```python
from build123d import *

# Parameters (mm, degrees)
SKETCH1_W                   = 72
SKETCH1_H                   = 35
BOSS_EXTRUDE1_DEPTH         = 6
CUT_EXTRUDE3_REACH          = 8
CUT_EXTRUDE4_REACH          = 8
SKETCH5_R                   = 1
FILLET1_R                   = 3
TAP_DRILL_FOR_M3_TAP1_D     = 2.5
TAP_DRILL_FOR_M3_TAP1_DEPTH = 10
TAP_DRILL_FOR_M3_TAP1_TIP   = 0.751075774
TAP_DRILL_FOR_M3_TAP2_D     = 2.5
TAP_DRILL_FOR_M3_TAP2_DEPTH = 10
TAP_DRILL_FOR_M3_TAP2_TIP   = 0.751075774


with BuildPart() as part:
    # Sketch1 → Boss-Extrude1 (new body)
    with BuildSketch(Plane(origin=(0, 0, 0), x_dir=(1, 0, 0), z_dir=(0, 1, 0))):
        with Locations((36, 17.5)):
            Rectangle(SKETCH1_W, SKETCH1_H)
    extrude(amount=BOSS_EXTRUDE1_DEPTH)

    # Sketch4 → Cut-Extrude3 (cut, up to next)
    with BuildSketch(Plane(origin=(0, 6, 0), x_dir=(1, 0, 0), z_dir=(0, 1, 0)), mode=Mode.PRIVATE) as cut_extrude3_sk1:
        Polygon((15, 0), (57, 0), (52.669872981, 7.5), (19.330127019, 7.5), align=None)
    cut_extrude3_tool1 = extrude(cut_extrude3_sk1.sketch, amount=-CUT_EXTRUDE3_REACH, mode=Mode.PRIVATE) & part.part
    add(cut_extrude3_tool1.solids().sort_by_distance((36, 6, -3.606313))[0], mode=Mode.SUBTRACT)

    # Sketch5 → Cut-Extrude4 (cut, up to next)
    with BuildSketch(Plane(origin=(0, 6, 0), x_dir=(1, 0, 0), z_dir=(0, 1, 0)), mode=Mode.PRIVATE) as cut_extrude4_sk1:
        with Locations((27, 12.5)):
            Circle(SKETCH5_R)
    cut_extrude4_tool1 = extrude(cut_extrude4_sk1.sketch, amount=-CUT_EXTRUDE4_REACH, mode=Mode.PRIVATE) & part.part
    add(cut_extrude4_tool1.solids().sort_by_distance((27, 6, -12.5))[0], mode=Mode.SUBTRACT)
    # Sketch5 → Cut-Extrude4 (cut, up to next)
    with BuildSketch(Plane(origin=(0, 6, 0), x_dir=(1, 0, 0), z_dir=(0, 1, 0)), mode=Mode.PRIVATE) as cut_extrude4_sk2:
        with Locations((45, 12.5)):
            Circle(SKETCH5_R)
    cut_extrude4_tool2 = extrude(cut_extrude4_sk2.sketch, amount=-CUT_EXTRUDE4_REACH, mode=Mode.PRIVATE) & part.part
    add(cut_extrude4_tool2.solids().sort_by_distance((45, 6, -12.5))[0], mode=Mode.SUBTRACT)
    # Sketch5 → Cut-Extrude4 (cut, up to next)
    with BuildSketch(Plane(origin=(0, 6, 0), x_dir=(1, 0, 0), z_dir=(0, 1, 0)), mode=Mode.PRIVATE) as cut_extrude4_sk3:
        with Locations((45, 31.5)):
            Circle(SKETCH5_R)
    cut_extrude4_tool3 = extrude(cut_extrude4_sk3.sketch, amount=-CUT_EXTRUDE4_REACH, mode=Mode.PRIVATE) & part.part
    add(cut_extrude4_tool3.solids().sort_by_distance((45, 6, -31.5))[0], mode=Mode.SUBTRACT)
    # Sketch5 → Cut-Extrude4 (cut, up to next)
    with BuildSketch(Plane(origin=(0, 6, 0), x_dir=(1, 0, 0), z_dir=(0, 1, 0)), mode=Mode.PRIVATE) as cut_extrude4_sk4:
        with Locations((27, 31.5)):
            Circle(SKETCH5_R)
    cut_extrude4_tool4 = extrude(cut_extrude4_sk4.sketch, amount=-CUT_EXTRUDE4_REACH, mode=Mode.PRIVATE) & part.part
    add(cut_extrude4_tool4.solids().sort_by_distance((27, 6, -31.5))[0], mode=Mode.SUBTRACT)

    # Fillet1
    fillet1_edges = [part.edges().sort_by_distance(p)[0] for p in [
        (15, 3, 0),
        (19.330127019, 3, -7.5),
        (52.669872981, 3, -7.5),
        (57, 3, 0),
    ]]
    fillet(fillet1_edges, radius=FILLET1_R)

    # Tap Drill for M3 Tap1
    with Locations(Plane.ZY):
        with Locations((-30, 3), (-5, 3)):
            Hole(TAP_DRILL_FOR_M3_TAP1_D / 2, depth=TAP_DRILL_FOR_M3_TAP1_DEPTH)
            with Locations((0, 0, -(TAP_DRILL_FOR_M3_TAP1_DEPTH + TAP_DRILL_FOR_M3_TAP1_TIP / 2))):  # 118° drill point
                Cone(0, TAP_DRILL_FOR_M3_TAP1_D / 2, TAP_DRILL_FOR_M3_TAP1_TIP, mode=Mode.SUBTRACT)

    # Tap Drill for M3 Tap2
    with Locations(Plane(origin=(72, 0, 0), x_dir=(0, 0, -1), z_dir=(1, 0, 0))):
        with Locations((5, 3), (30, 3)):
            Hole(TAP_DRILL_FOR_M3_TAP2_D / 2, depth=TAP_DRILL_FOR_M3_TAP2_DEPTH)
            with Locations((0, 0, -(TAP_DRILL_FOR_M3_TAP2_DEPTH + TAP_DRILL_FOR_M3_TAP2_TIP / 2))):  # 118° drill point
                Cone(0, TAP_DRILL_FOR_M3_TAP2_D / 2, TAP_DRILL_FOR_M3_TAP2_TIP, mode=Mode.SUBTRACT)


solid = part.part
```
Can you work these out from the model? Positions are in its coordinate system, mm. A direction names the side the tool comes from. Coordinates: 2 decimals unless noted, no trailing zeros. Loops run counter-clockwise (first coordinate to the right, second up) from the corner with the lowest first, then second, coordinate; pieces in that order, holes last. Notation, with made-up numbers: (47.5, 28.25) - (77.5, 28.25) arc R14 ccw to (77.5, 50.25) - close; hole circle Ø5 at (0.5, 52). An arc over 180 degrees is marked (long way). Use a Markdown table: item, result.
Item 1: Will these pins go through, and if not, where does the flat tip stop? pin 1 (2 mm diameter, centred on y = 3, z = -5, fed in from -X); pin 2 (2 mm diameter, centred on y = 3, z = -30, fed in from +X); pin 3 (1.6 mm diameter, centred on x = 27, z = -12.5, fed in from -Y).
Numbers:
| item | result |
|---|---|
| pin 1 | stops at x = 10.15 |
| pin 2 | stops at x = 61.85 |
| pin 3 | passes through |
Item 2: I want a section at C-C on x = 6. Please give me the cut outline in (y, z).
Numbers:
| item | result |
|---|---|
| outline | (0, -35) - (6, -35) - (6, 0) - (0, 0) - close; hole circle Ø2.5 at (3, -30); hole circle Ø2.5 at (3, -5) |
Item 3: I want a section at A-A on z = -12.5. Please give me the cut outline in (x, y).
Numbers:
| item | result |
|---|---|
| outline | (0, 0) - (26, 0) - (26, 6) - (0, 6) - close; (28, 0) - (44, 0) - (44, 6) - (28, 6) - close; (46, 0) - (72, 0) - (72, 6) - (46, 6) - close |
Item 4: For faces 4 (the face through (57.25, 2.96, -0.39)), 5 (the face through (5.07, 3.38, -31.19)), 6 (the face through (66.93, 3.845, -5.921)), 7 (the face through (72, 3, -17)), which set-ups out of +Z, -Z, +X, -X, +Y, -Y let a thin tool reach every point of the face, with its end or its side?
Numbers:
| item | result |
|---|---|
| face 4 | +Z, +Y, -Y |
| face 5 | -X |
| face 6 | +X |
| face 7 | +Z, -Z, +X, +Y, -Y |
Item 5: I want a section at B-B on x = 45. Please give me the cut outline in (y, z), and give its area (3 significant figures).
Numbers:
| item | result |
|---|---|
| outline | (0, -35) - (6, -35) - (6, -32.5) - (0, -32.5) - close; (0, -30.5) - (6, -30.5) - (6, -13.5) - (0, -13.5) - close; (0, -11.5) - (6, -11.5) - (6, -7.5) - (0, -7.5) - close |
| area | 141 mm2 |
Item 6: If I drill on probe 1 along Z at (x, y) = (65, 3); probe 2 along Z at (x, y) = (45, 4.75); probe 3 along X at (y, z) = (3.2, -12.5), over which ranges is the centre line in solid material (lowest first)? Write a range as from..to.
Numbers:
| item | result |
|---|---|
| probe 1 | z = -35..-31.25, -28.75..-6.25, -3.75..0 |
| probe 2 | z = -35..-32.5, -30.5..-13.5, -11.5..-7.5 |
| probe 3 | x = 0..26, 28..44, 46..72 |
Item 7: We'd pull the mould along Y, two halves only. Please class faces 1 (the face through (65, 3, 0)), 2 (the face through (35, 0, -18)), 3 (the face through (61.38, 2.92, -30.2)): released by +Y, released by -Y, zero draft, split by the parting line, or undercut.
Numbers:
| item | result |
|---|---|
| face 1 | zero draft |
| face 2 | released by -Y |
| face 3 | undercut |
